Design review of the part shown in the three views and the two pictorial views. Dimensions are in mm from the part's minimum x, y and z. A direction names the side the tool comes from. Give positions to 0.01 mm unless a question says otherwise; leave off trailing zeros. Loops run counter-clockwise (first coordinate to the right, second up) from the corner with the lowest first, then second, coordinate; pieces in that order, holes last. Notation, with made-up numbers: (79, 28.5) - (84, 28.5) arc R20 ccw to (84, 35.5) - close; hole circle Ø1 at (39.25, 12). An arc over 180 degrees is marked (long way). Answer as a JSON object with one key per item and string values.
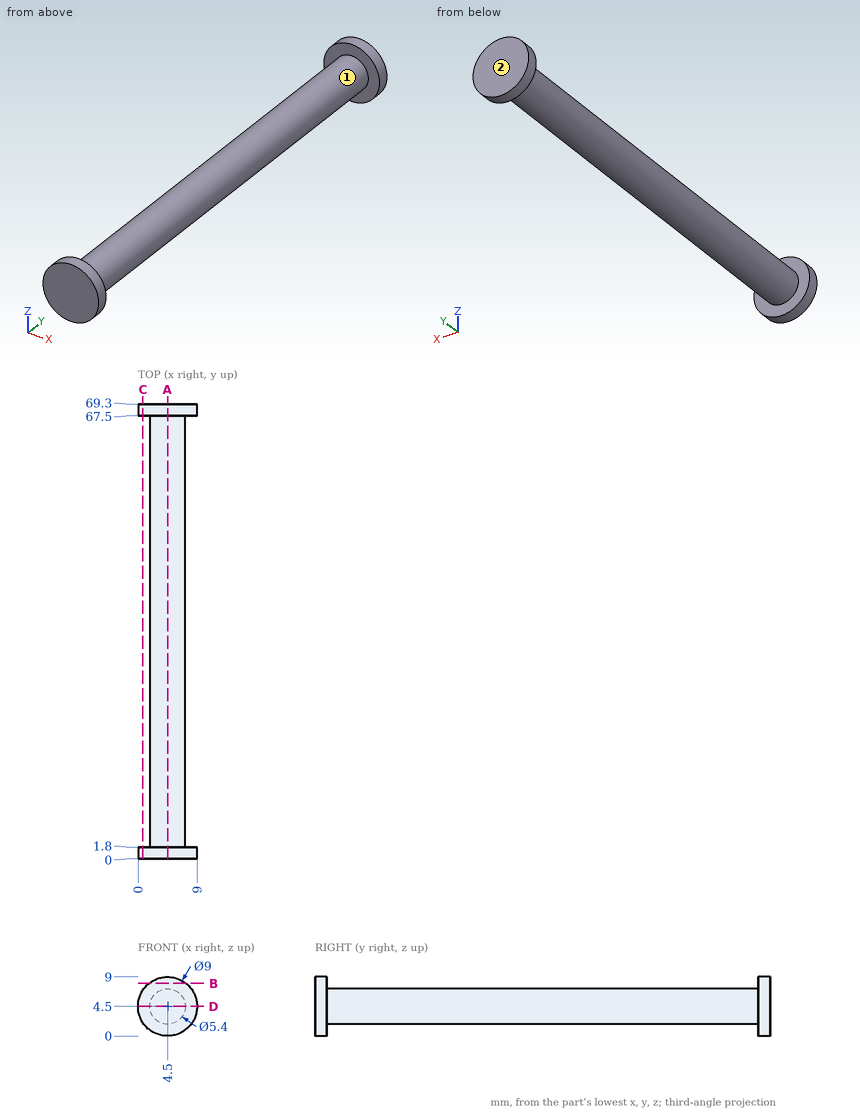
Q1. For the marked faces 1 and 2, list the 3-axis set-ups (+Z, -Z, +X, -X, +Y, -Y) from which the entire face can be reached by the end or side of a thin tool; tool diameter is ignored.
Results:
{"face 1": "none", "face 2": "+Z, -Z, +X, -X, +Y"}
Q2. Consider section B-B, the plane z = 8. State the section outline as (x, y) points.
Results:
{"outline": "(1.67, 0) - (7.33, 0) - (7.33, 1.8) - (1.67, 1.8) - close; (1.67, 67.5) - (7.33, 67.5) - (7.33, 69.3) - (1.67, 69.3) - close"}
Q3. Consider section D-D, the plane z = 4.5. State the section outline as (x, y) points.
Results:
{"outline": "(0, 0) - (9, 0) - (9, 1.8) - (7.2, 1.8) - (7.2, 67.5) - (9, 67.5) - (9, 69.3) - (0, 69.3) - (0, 67.5) - (1.8, 67.5) - (1.8, 1.8) - (0, 1.8) - close"}
Q4. To check wall thickness, follow probe 1 along Y at (x, z) = (1, 4); probe 2 along Z at (x, y) = (4.5, 34); probe 3 along Z at (x, y) = (6.5, 34). State the ranges of each line that lie inside material, in increasing order. Write a range as [from, to].
Results:
{"probe 1": "y = [0, 1.8], [67.5, 69.3]", "probe 2": "z = [1.8, 7.2]", "probe 3": "z = [2.69, 6.31]"}
Q5. Clearance check with flat-ended pins moving along their axes: pin 1 Ø4 at (y, z) = (38, 4) entering from +X; pin 2 Ø3 at (x, y) = (6, 19.5) entering from -Z; pin 3 Ø1 at (y, z) = (22, 7) entering from -X; pin 4 Ø4.5 at (x, z) = (4.5, 3) entering from -Y. State where each tip first meets the part, or that it passes through.
Results:
{"pin 1": "stops at x = 7.2", "pin 2": "stops at z = 1.8", "pin 3": "stops at x = 2.69", "pin 4": "stops at y = 0"}
Q6. Consider section A-A, the plane x = 4.5. State the section outline as (y, z) points, plus the area to 3 significant figures.
Results:
{"outline": "(0, 0) - (1.8, 0) - (1.8, 1.8) - (67.5, 1.8) - (67.5, 0) - (69.3, 0) - (69.3, 9) - (67.5, 9) - (67.5, 7.2) - (1.8, 7.2) - (1.8, 9) - (0, 9) - close", "area": "387 mm^2"}
Q7. Consider section C-C, the plane x = 0.75. State the section outline as (y, z) points, plus the area to 3 significant figures.
Results:
{"outline": "(0, 2.01) - (1.8, 2.01) - (1.8, 6.99) - (0, 6.99) - close; (67.5, 2.01) - (69.3, 2.01) - (69.3, 6.99) - (67.5, 6.99) - close", "area": "17.9 mm^2"}
